```python
from build123d import *

# Parameters (mm, degrees)
EXTRUDE_THIN2_DEPTH     = 65
CUT_EXTRUDE3_DEPTH      = 186.389784583
CUT_EXTRUDE3_DEPTH_BACK = 186.389784583
CUT_EXTRUDE4_DEPTH      = 186.389784583
CUT_EXTRUDE4_DEPTH_BACK = 186.389784583


with BuildPart() as part:
    # Sketch1 → Extrude-Thin2 (new body)
    with BuildSketch(Plane(origin=(0, 0, 0), x_dir=(0, 0, -1), z_dir=(1, 0, 0))):
        with BuildLine():
            Line((173.642321834, 9.797958971), (-66.357678166, 28.050095))
            ThreePointArc((-66.357678166, 28.050095), (-91.137548283, 20.841238484), (-106.357678166, 0))
            Line((-106.357678166, 0), (-107.789658514, 0.446578419))
            ThreePointArc((-107.789658514, 0.446578419), (-91.989308326, 22.075999038), (-66.266563175, 29.547497166))
            Line((-66.266563175, 29.547497166), (173.756069218, 11.293639931))
            Line((173.756069218, 11.293639931), (173.642321834, 9.797958971))
        make_face()
    extrude(amount=EXTRUDE_THIN2_DEPTH)

    # Sketch2 → Cut-Extrude3 (cut, two sides: drawn at the far end of the back side and taken through both)
    with BuildSketch(Plane(origin=(0, 24.366956586, -1.853120859), x_dir=(1, 0, 0), z_dir=(0, 0.9971206396362033, -0.07583158979929651)).offset(-CUT_EXTRUDE3_DEPTH_BACK)):
        Polygon((93.231917992, 749.14649506), (20, 172.399348209), (0, 14.886842005), (-73.231917992, -561.860304846), (-1226.726211693, -415.396468862), (-1060.262375709, 895.610331043), align=None)
    extrude(amount=CUT_EXTRUDE3_DEPTH + CUT_EXTRUDE3_DEPTH_BACK, mode=Mode.SUBTRACT)

    # Sketch4 → Cut-Extrude4 (cut, two sides: drawn at the far end of the back side and taken through both)
    with BuildSketch(Plane(origin=(0, 24.366956586, -1.853120859), x_dir=(1, 0, 0), z_dir=(0, 0.9971206396362033, -0.07583158979929651)).offset(-CUT_EXTRUDE4_DEPTH_BACK)):
        Polygon((-28.231917992, 749.14649506), (45, 172.399348209), (65, 14.886842005), (138.231917992, -561.860304846), (1291.726211693, -415.396468862), (1125.262375709, 895.610331043), align=None)
    extrude(amount=CUT_EXTRUDE4_DEPTH + CUT_EXTRUDE4_DEPTH_BACK, mode=Mode.SUBTRACT)


solid = part.part
```
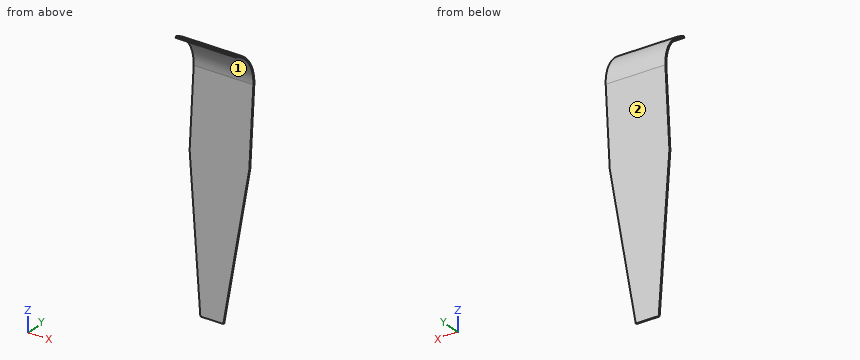
Build history of the part. All positions in model axes, mm. Face numbers are marked on the shaded views. Give positions to 0.01 mm unless a question says otherwise; leave off trailing zeros. Loops run counter-clockwise (first coordinate to the right, second up) from the corner with the lowest first, then second, coordinate; pieces in that order, holes last. Notation, with made-up numbers: (-37, -30) - (-21, -30) arc R29 ccw to (-21, -2) - close; hole circle Ø7 at (60, 75). An arc over 180 degrees is marked (long way). Use a Markdown table: item, result.
(1) Drop flat-ended pins along their axis: pin 1 Ø10 at (x, z) = (16, -41) entering from +Y; pin 2 Ø8 at (y, z) = (11, -131.5) entering from +X; pin 3 Ø4 at (x, z) = (52.5, 46.5) entering from +Y; pin 4 Ø5 at (y, z) = (22, -67.5) entering from +X. Give the stop position or say it passes through.
Taken from the geometry:
| item | result |
|---|---|
| pin 1 | y = 21.77 |
| pin 2 | x = 50.79 |
| pin 3 | y = 28.2 |
| pin 4 | through |
(2) Wall check: line 1 along Y through (x, z) = (7, 67.5); line 2 along Y through (x, z) = (20, -136); line 3 along X through (y, z) = (18.5, -64). Give the ranges that are in metal, low to high.
Taken from the geometry:
| item | result |
|---|---|
| line 1 | 28.09 to 29.59 |
| line 2 | 12.66 to 14.17 |
| line 3 | 6.03 to 58.97 |
(3) Band-saw the part on C-C (y = 4). Give the cut face in (x, z), and give its area (3 significant figures).
Taken from the geometry:
| item | result |
|---|---|
| outline | (0, 104.87) - (65, 104.87) - (65, 106.5) - (0, 106.5) - close |
| area | 106 mm2 |
(4) Band-saw the part on B-B (x = 42). Give the cut face in (y, z).
Taken from the geometry:
| item | result |
|---|---|
| outline | (0, 106.36) arc R40 cw to (28.05, 66.36) - (9.8, -173.64) - (11.29, -173.76) - (29.55, 66.27) arc R41.5 ccw to (0.45, 107.79) - close |
(5) Band-saw the part on A-A (y = 16.5). Give the cut face in (x, z), and give its area (3 significant figures).
Taken from the geometry:
| item | result |
|---|---|
| outline | (0, 96.33) - (65, 96.33) - (65, 98.42) - (0, 98.42) - close; (8.78, -85.52) - (11.28, -105.3) - (53.72, -105.3) - (56.22, -85.52) - close |
| area | 1,020 mm2 |
(6) Pull direction Z, two halves, no side cores. Call the marked faces 1 and 2: +Z half, -Z half, draft (parallel to the pull), parting line (faces both ways), or undercut.
Taken from the geometry:
| item | result |
|---|---|
| face 1 | undercut |
| face 2 | -Z half |
(7) Band-saw the part on D-D (z = 59.5). Give the cut face in (x, y), and give its area (3 significant figures).
Taken from the geometry:
| item | result |
|---|---|
| outline | (0, 27.53) - (65, 27.53) - (65, 29.03) - (0, 29.03) - close |
| area | 97.8 mm2 |
